```python
from build123d import *

# Parameters (mm, degrees)
ESBO_O1_W                               = 125
ESBO_O1_H                               = 125
RESSALTO_EXTRUS_O1_DEPTH                = 5
ESBO_O2_R                               = 17.5
CORTE_EXTRUS_O1_DEPTH                   = 89.529656048
BROCA_DE_ROSQUEAR_PARA_TARRAXA_DE_M51_D = 4.2
FURO_COM_FOLGA_DE_M51_D                 = 5.3


with BuildPart() as part:
    # Esboço1 → Ressalto-extrusão1 (new body)
    with BuildSketch(Plane(origin=(0, 0, 0), x_dir=(1, 0, 0), z_dir=(0, 1, 0))):
        Rectangle(ESBO_O1_W, ESBO_O1_H)
    extrude(amount=RESSALTO_EXTRUS_O1_DEPTH)

    # Esboço2 → Corte-extrusão1 (cut, through all)
    with BuildSketch(Plane(origin=(0, 5, 0), x_dir=(1, 0, 0), z_dir=(0, 1, 0))):
        with Locations(Location((0, 0, 0), (0, 0, 270))):
            Circle(ESBO_O2_R)
    extrude(amount=-CORTE_EXTRUS_O1_DEPTH, mode=Mode.SUBTRACT)

    # Broca de rosquear para tarraxa de M51 (through all)
    with Locations(Plane(origin=(0, 5, 0), x_dir=(1, 0, 0), z_dir=(0, 1, 0))):
        with Locations((28.284271247, 28.284271247), (28.284271247, -28.284271247), (-28.284271247, -28.284271247), (-28.284271247, 28.284271247)):
            Hole(BROCA_DE_ROSQUEAR_PARA_TARRAXA_DE_M51_D / 2)

    # Furo com folga de M51 (through all)
    with Locations(Plane(origin=(0, 5, 0), x_dir=(1, 0, 0), z_dir=(0, 1, 0))):
        with Locations((-50, -50), (-50, 50), (50, 50), (50, -50)):
            Hole(FURO_COM_FOLGA_DE_M51_D / 2)


solid = part.part
```
Can you work these out from the model? Positions are in its coordinate system, mm. Coordinates: 2 decimals unless noted, no trailing zeros. Order: outer loops, then holes, each group sorted by start corner. A loop starts at its lowest first (then second) coordinate and runs counter-clockwise, first axis right, second up.
1. If we section it at C-C (z = 50): Please give me the cut outline in (x, y), then the cut area to 3 significant figures.
2. If we section it at B-B (x = -50): Please give me the cut outline in (y, z), then the cut area to 3 significant figures.
3. If we section it at D-D (x = 0): Please give me the cut outline in (y, z).
4. Thinking about a two-plate mould opening in Z: for faces 1 (the face through (-1, 2, -62.5)), 2 (the face through (62.5, 2, 1)), 3 (the face through (50.34, 2.47, 47.37)), which applies, +Z half, -Z half, draft (parallel to the pull), parting line (faces both ways), or undercut?
5. I'm going to push a flat-ended pin straight in: pin 1 (3 mm diameter, centred on x = -50, z = 50, fed in from -Y). Where does the tip first touch, or does it pass through?
6. If we section it at A-A (z = 10.5): Please give me the cut outline in (x, y), then the cut area to 3 significant figures.
7. I need wall thicknesses on line 1 (Z direction, x = 50, y = 2.3); line 2 (X direction, y = 3.1, z = -28). Which ranges of each line are inside material? Lowest first, please.
Entries:
1. outline: (-62.5, 0) - (-52.65, 0) - (-52.65, 5) - (-62.5, 5) - close; (-47.35, 0) - (47.35, 0) - (47.35, 5) - (-47.35, 5) - close; (52.65, 0) - (62.5, 0) - (62.5, 5) - (52.65, 5) - close
1. area: 572 mm2
2. outline: (0, -62.5) - (5, -62.5) - (5, -52.65) - (0, -52.65) - close; (0, -47.35) - (5, -47.35) - (5, 47.35) - (0, 47.35) - close; (0, 52.65) - (5, 52.65) - (5, 62.5) - (0, 62.5) - close
2. area: 572 mm2
3. outline: (0, -62.5) - (5, -62.5) - (5, -17.5) - (0, -17.5) - close; (0, 17.5) - (5, 17.5) - (5, 62.5) - (0, 62.5) - close
4. face 1: -Z half
4. face 2: draft
4. face 3: undercut
5. pin 1: passes through
6. outline: (-62.5, 0) - (-14, 0) - (-14, 5) - (-62.5, 5) - close; (14, 0) - (62.5, 0) - (62.5, 5) - (14, 5) - close
6. area: 485 mm2
7. line 1: z = -62.5 to -52.65, -47.35 to 47.35, 52.65 to 62.5
7. line 2: x = -62.5 to -30.36, -26.2 to 26.2, 30.36 to 62.5
